Geometry: see drawing. Coordinates: mm, zero at the bounding-box minimum. A direction names the side the tool comes from. Coordinates: 2 decimals unless noted, no trailing zeros. Order: outer loops, then holes, each group sorted by start corner. A loop starts at its lowest first (then second) coordinate and runs counter-clockwise, first axis right, second up. Notation, with made-up numbers: (26, -26) - (68, -26) arc R28 cw to (68, 1) - close; hole circle Ø6 at (-4, -7.5). An arc over 180 degrees is marked (long way). Use a Markdown table: item, result. Add a question column.
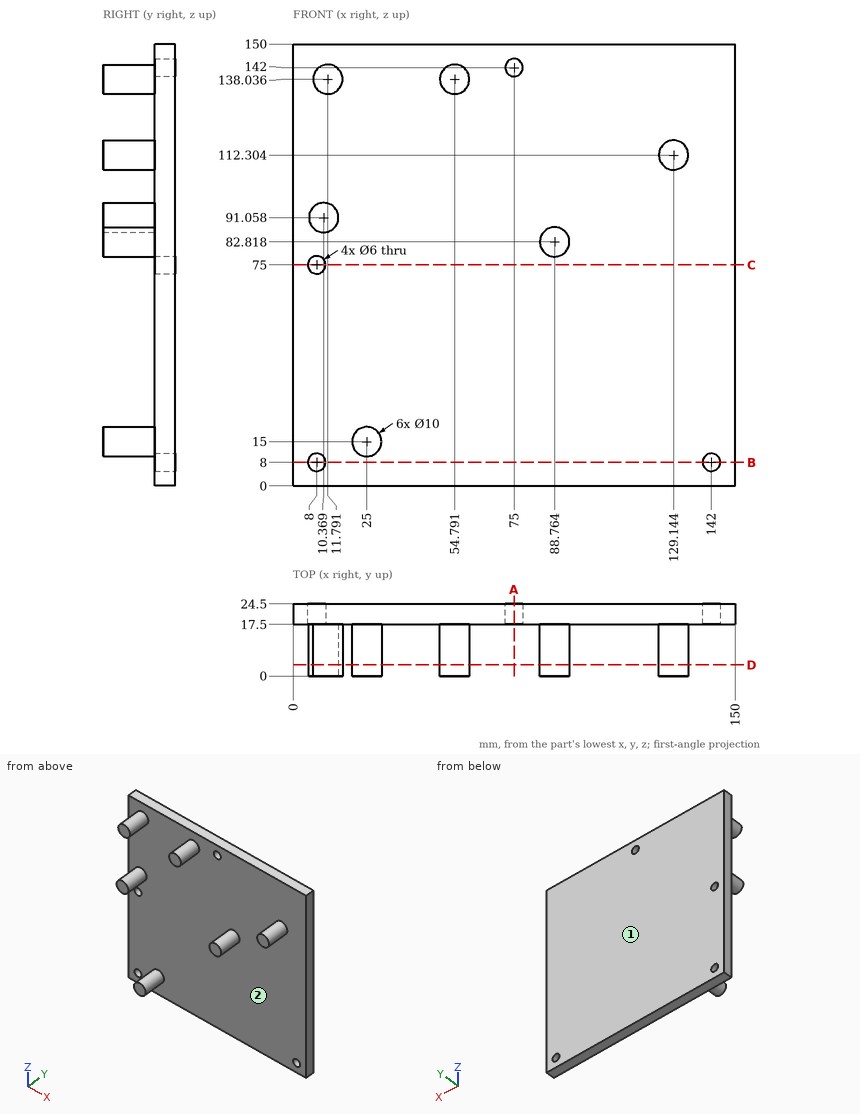
1) Section query A-A (x = 75). Return the cut outline in (y, z), and give its area (3 significant figures).
2) Line query: line 1 (Z direction, x = 8, y = 19); line 2 (Z direction, x = 75, y = 21.5); line 3 (Z direction, x = 142, y = 21). Output: solid intervals per line, ascending. Write a range as from..to.
3) Section query C-C (z = 75). Return the cut outline in (x, y).
4) Section query D-D (y = 3.75). Return the cut outline in (x, z) (1 decimal), and give its area (3 significant figures).
5) Section query B-B (z = 8). Return the cut outline in (x, y), and give its area (3 significant figures).
6) First-contact query: pin 1 (2 mm diameter, centred on x = 92.5, z = 117.5, fed in from -Y); pin 2 (1.5 mm diameter, centred on y = 18.5, z = 45.5, fed in from -X). Flat tips, straight axial feed; report the tip coordinate or a pass-through.
7) Access query for the marked faces 1 and 2. Directions: +Z, -Z, +X, -X, +Y, -Y. A direction counts if a zero-diameter tool reaches every point of the face in a straight line with its end or side. Return the directions, or none.
From the geometry:
| question | item | result |
|---|---|---|
| 1 | outline | (17.5, 0) - (24.5, 0) - (24.5, 139) - (17.5, 139) - close; (17.5, 145) - (24.5, 145) - (24.5, 150) - (17.5, 150) - close |
| 1 | area | 1,010 mm^2 |
| 2 | line 1 | z = 0..5, 11..72, 78..150 |
| 2 | line 2 | z = 0..139, 145..150 |
| 2 | line 3 | z = 0..5, 11..150 |
| 3 | outline | (0, 17.5) - (5, 17.5) - (5, 24.5) - (0, 24.5) - close; (11, 17.5) - (150, 17.5) - (150, 24.5) - (11, 24.5) - close |
| 4 | outline | circle Ø10 at (10.4, 91.1); circle Ø10 at (11.8, 138); circle Ø10 at (25, 15); circle Ø10 at (54.8, 138); circle Ø10 at (88.8, 82.8); circle Ø10 at (129.1, 112.3) |
| 4 | area | 471 mm^2 |
| 5 | outline | (0, 17.5) - (5, 17.5) - (5, 24.5) - (0, 24.5) - close; (11, 17.5) - (139, 17.5) - (139, 24.5) - (11, 24.5) - close; (145, 17.5) - (150, 17.5) - (150, 24.5) - (145, 24.5) - close |
| 5 | area | 966 mm^2 |
| 6 | pin 1 | stops at y = 17.5 |
| 6 | pin 2 | stops at x = 0 |
| 7 | face 1 | +Z, -Z, +X, -X, +Y |
| 7 | face 2 | -Y |
